Answer from the drawing. Dimensions are ordinates in mm from the lowest x, y and z of the part. A direction names the side the tool comes from. Coordinates: 2 decimals unless noted, no trailing zeros. Write each loop counter-clockwise with the first axis right and the second up, starting at its lowest first coordinate (ties: lowest second). Pieces come first, ordered by that corner, then holes. Notation, with made-up numbers: (-22, 73.25) -> (2, 73.25) arc R19 cw to (2, 101.25) -> close; hole circle Ø10 at (-4, 17.5). An arc over 180 degrees is marked (long way). Return JSON: item names as keys, results as strings.
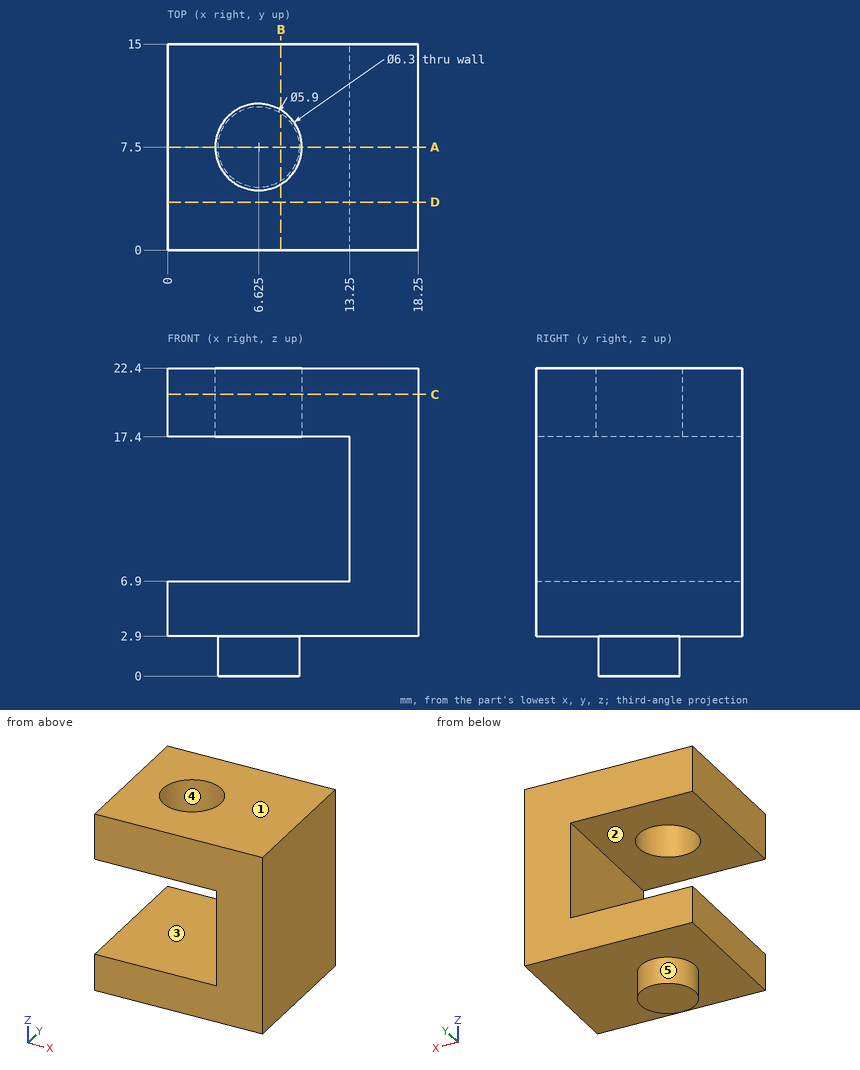
1. A tool of negligible diameter and unlimited length cuts with its end or side. For the marked faces 1 and 2, from which of +Z, -Z, +X, -X, +Y, -Y can it reach the whole face along a straight path? Write none if from no direction.
Taken from the geometry:
{"face 1": "+Z, +X, -X, +Y, -Y", "face 2": "-X, +Y, -Y"}
2. The part is cut by section C-C (z = 20.5). Determine the outline of the cut face in (x, y) (3 decimals), then the cut area to 3 significant figures.
Taken from the geometry:
{"outline": "(0, 0) -> (18.25, 0) -> (18.25, 15) -> (0, 15) -> close; hole circle Ø6.3 at (6.625, 7.5)", "area": "243 mm2"}
3. Flat-ended cylindrical pins translate along their axes: pin 1 Ø4 at (x, z) = (9, 14) entering from +Y; pin 2 Ø3 at (x, y) = (12.5, 3) entering from -Z; pin 3 Ø1 at (y, z) = (6.5, 11.5) entering from -X. Find the tip coordinate at first contact, or state that the pin passes through.
Taken from the geometry:
{"pin 1": "passes through", "pin 2": "stops at z = 2.9", "pin 3": "stops at x = 13.25"}
4. The part is cut by section B-B (x = 8.25). Determine the outline of the cut face in (y, z).
Taken from the geometry:
{"outline": "(0, 2.9) -> (5.04, 2.9) -> (5.04, 0) -> (9.96, 0) -> (9.96, 2.9) -> (15, 2.9) -> (15, 6.9) -> (0, 6.9) -> close; (0, 17.4) -> (4.8, 17.4) -> (4.8, 22.4) -> (0, 22.4) -> close; (10.2, 17.4) -> (15, 17.4) -> (15, 22.4) -> (10.2, 22.4) -> close"}
5. The part is cut by section D-D (y = 3.5). Determine the outline of the cut face in (x, z).
Taken from the geometry:
{"outline": "(0, 2.9) -> (18.25, 2.9) -> (18.25, 22.4) -> (0, 22.4) -> (0, 17.4) -> (13.25, 17.4) -> (13.25, 6.9) -> (0, 6.9) -> close"}
6. Consider L1, parallel to Z at x = 11, y = 3.75; L2, parallel to X at y = 7, z = 14.5; L3, parallel to Z at x = 14.5, y = 2.5. Determine where each line is inside the solid, lowest interval first.
Taken from the geometry:
{"L1": "z = 2.9 to 6.9, 17.4 to 22.4", "L2": "x = 13.25 to 18.25", "L3": "z = 2.9 to 22.4"}
7. The part is cut by section A-A (y = 7.5). Determine the outline of the cut face in (x, z) (3 decimals).
Taken from the geometry:
{"outline": "(0, 2.9) -> (3.675, 2.9) -> (3.675, 0) -> (9.575, 0) -> (9.575, 2.9) -> (18.25, 2.9) -> (18.25, 22.4) -> (9.775, 22.4) -> (9.775, 17.4) -> (13.25, 17.4) -> (13.25, 6.9) -> (0, 6.9) -> close; (0, 17.4) -> (3.475, 17.4) -> (3.475, 22.4) -> (0, 22.4) -> close"}
8. For a pull along X with two mould halves and no side action, classify the marked faces 3, 4 and 5 as +X half, -X half, draft (parallel to the pull), parting line (faces both ways), or undercut.
Taken from the geometry:
{"face 3": "draft", "face 4": "undercut", "face 5": "parting line"}
